from build123d import *

# Parameters (mm, degrees)
SKETCH_W            = 86.36
SKETCH_H            = 113.03
PAD_DEPTH           = 10
SKETCH001_R         = 1.6
POCKET_DEPTH        = 1
POCKET001_DEPTH     = 9
CHAMFER_SIZE        = 3
FILLET_R            = 6
FILLET_FACE23_R     = 1.6
POCKET002_DEPTH     = 9.001
POCKET002_FACE25_R  = 1.6
POCKET003_DEPTH     = 9.001
SKETCH003_R         = 2.8
POCKET005_DEPTH     = 4
POCKET006_DEPTH     = 10.001
POCKET006_FACE37_R  = 1.6
POCKET007_DEPTH     = 9.0010001
POCKET007_FACE6_R   = 1.6
POCKET008_DEPTH     = 4.5
CHAMFER001_SIZE     = 3
CHAMFER001_FACE10_W = 66.9783844647
CHAMFER001_FACE10_H = 4.5
POCKET009_DEPTH     = 2.5
CHAMFER002_SIZE     = 1


with BuildPart() as part:
    # Sketch → Pad (new body)
    with BuildSketch(Plane.XY):
        Rectangle(SKETCH_W, SKETCH_H)
    extrude(amount=PAD_DEPTH)

    # Sketch001 (on Face6 of Pad) → Pocket (cut)
    with BuildSketch(Plane.XY.offset(10)):
        with Locations((-39.37, -52.705)):
            Circle(SKETCH001_R)
        with Locations((39.37, -52.705)):
            Circle(SKETCH001_R)
        with Locations((39.37, 52.705)):
            Circle(SKETCH001_R)
    extrude(amount=-POCKET_DEPTH, mode=Mode.SUBTRACT)

    # Sketch002 (on Face5 of Pocket) → Pocket001 (cut)
    with BuildSketch(Plane.XY.offset(10)):
        with BuildLine():
            Line((-38.18, 56.515), (34.734927185, 56.515))
            ThreePointArc((34.734927185, 56.515), (33.7166110056, 50.695225665), (38.18, 46.8241922324))
            Line((38.18, -46.8241922324), (38.18, 46.8241922324))
            ThreePointArc((38.18, -46.8241922324), (35.1273593129, -48.4623593129), (33.4891922324, -51.515))
            Line((-33.4891922324, -51.515), (33.4891922324, -51.515))
            ThreePointArc((-33.4891922324, -51.515), (-35.1273593129, -48.4623593129), (-38.18, -46.8241922324))
            Line((-38.18, -46.8241922324), (-38.18, 56.515))
        make_face()
    extrude(amount=-POCKET001_DEPTH, mode=Mode.SUBTRACT)

    # Chamfer
    chamfer_edges = [part.edges().sort_by_distance(p)[0] for p in [
        (43.18, 0, 0),
        (0, -56.515, 0),
        (-43.18, 0, 0),
    ]]
    chamfer(chamfer_edges, length=CHAMFER_SIZE)

    # Fillet
    fillet_edges = [part.edges().sort_by_distance(p)[0] for p in [
        (43.18, 0, 3),
        (0, -56.515, 3),
        (-43.18, 0, 3),
    ]]
    fillet(fillet_edges, radius=FILLET_R)

    # Fillet Face23 → Pocket002 (cut, through all)
    with BuildSketch(Plane(origin=(39.37, 52.705, 9), x_dir=(0, 1, 0), z_dir=(0, 0, 1))):
        Circle(FILLET_FACE23_R)
    extrude(amount=-POCKET002_DEPTH, mode=Mode.SUBTRACT)

    # Pocket002 Face25 → Pocket003 (cut, through all)
    with BuildSketch(Plane(origin=(39.37, -52.705, 9), x_dir=(0, 1, 0), z_dir=(0, 0, 1))):
        Circle(POCKET002_FACE25_R)
    extrude(amount=-POCKET003_DEPTH, mode=Mode.SUBTRACT)

    # Sketch003 → Pocket005 (cut)
    with BuildSketch(Plane(origin=(0, 0, 0), x_dir=(1, 0, 0), z_dir=(0, 0, -1))):
        with Locations((-39.37, 52.705)):
            Circle(SKETCH003_R)
        with Locations((39.37, 52.705)):
            Circle(SKETCH003_R)
        with Locations((39.37, -52.705)):
            Circle(SKETCH003_R)
    extrude(amount=-POCKET005_DEPTH, mode=Mode.SUBTRACT)

    # Sketch004 (on Face4 of Pocket005) → Pocket006 (cut, through all)
    with BuildSketch(Plane(origin=(0, 0, 0), x_dir=(1, 0, 0), z_dir=(0, 0, -1))):
        Polygon((34.734927185, -56.515), (-43.18, -31.515), (-74.957912, -45.45311), (-56.152271, -90.823143), (38.876451, -98.385315), align=None)
    extrude(amount=-POCKET006_DEPTH, mode=Mode.SUBTRACT)

    # Pocket006 Face37 → Pocket007 (cut, through all)
    with BuildSketch(Plane(origin=(-39.37, -52.705, 9), x_dir=(0, 1, 0), z_dir=(0, 0, 1))):
        Circle(POCKET006_FACE37_R)
    extrude(amount=-POCKET007_DEPTH, mode=Mode.SUBTRACT)

    # Pocket007 Face6 → Pocket008 (cut)
    with BuildSketch(Plane(origin=(4.1610773178, -17.506602636, 10), x_dir=(0, 1, 0), z_dir=(0, 0, 1))):
        with BuildLine():
            Line((-39.008397364, 47.3410773178), (-39.008397364, -39.0189226822))
            Line((-39.008397364, -39.0189226822), (74.021602636, -39.0189226822))
            Line((74.021602636, -39.0189226822), (74.021602636, -30.5738498672))
            ThreePointArc((74.021602636, -30.5738498672), (68.201828301, -29.5555336878), (64.3307948684, -34.0189226822))
            Line((64.3307948684, -34.0189226822), (-29.3175895963, -34.0189226822))
            ThreePointArc((-29.3175895963, -34.0189226822), (-30.9557566768, -30.9662819951), (-34.008397364, -29.3281149145))
            Line((-34.008397364, -29.3281149145), (-34.008397364, 37.6502695502))
            ThreePointArc((-34.008397364, 37.6502695502), (-30.9557566768, 39.2884366307), (-29.3175895963, 42.3410773178))
            Line((-29.3175895963, 42.3410773178), (50.6259165271, 42.3410773178))
            Line((50.6259165271, 42.3410773178), (49.021602636, 47.3410773178))
            Line((49.021602636, 47.3410773178), (-39.008397364, 47.3410773178))
        make_face()
        with Locations((-35.198397364, -35.2089226822)):
            Circle(POCKET007_FACE6_R, mode=Mode.SUBTRACT)
        with Locations((70.211602636, -35.2089226822)):
            Circle(POCKET007_FACE6_R, mode=Mode.SUBTRACT)
        with Locations((-35.198397364, 43.5310773178)):
            Circle(POCKET007_FACE6_R, mode=Mode.SUBTRACT)
    extrude(amount=-POCKET008_DEPTH, mode=Mode.SUBTRACT)

    # Chamfer001
    chamfer001_edges = [part.edges().sort_by_distance(p)[0] for p in [
        (-38.18, -6.852439, 1),
        (38.18, 0, 1),
    ]]
    chamfer(chamfer001_edges, length=CHAMFER001_SIZE)

    # Chamfer001 Face10 → Pocket009 (cut)
    with BuildSketch(Plane(origin=(0, -51.515, 3.25), x_dir=(1, 0, 0), z_dir=(0, 1, 0))):
        Rectangle(CHAMFER001_FACE10_W, CHAMFER001_FACE10_H)
    extrude(amount=-POCKET009_DEPTH, mode=Mode.SUBTRACT)

    # Chamfer002
    chamfer002_edges = [part.edges().sort_by_distance(p)[0] for p in [
        (0, -54.015, 1),
    ]]
    chamfer(chamfer002_edges, length=CHAMFER002_SIZE)


solid = part.part
Here's how the part is built. I have some questions about the finished solid (model axes, mm). A direction names the side the tool comes from. Give positions to 0.01 mm unless a question says otherwise; leave off trailing zeros. Loops run counter-clockwise (first coordinate to the right, second up) from the corner with the lowest first, then second, coordinate; pieces in that order, holes last. Notation, with made-up numbers: (-0.5, 69) -> (11.5, 69) arc R11 ccw to (11.5, 88) -> close; hole circle Ø7 at (74, 53.25). An arc over 180 degrees is marked (long way). One line per item, written item: value.
Q1. Suppose I cut it at C-C on x = 14.5. Please give me the cut outline in (y, z) (3 decimals), then the cut area to 3 significant figures.
Answers follow:
outline: (-56.515, 5.485) arc R6 ccw to (-54.758, 1.243) -> (-53.515, 0) -> (50.022, 0) -> (50.022, 1) -> (-53.015, 1) -> (-54.015, 2) -> (-54.015, 5.5) -> (-56.515, 5.5) -> close
area: 113 mm^2
Q2. We'd pull the mould along X, two halves only. Please class faces 5 (the face through (37.15, -51, 2.42)), 6 (the face through (-12.698, 41.296, 0.496)), 7 (the face through (41, -17, 5.5)): pulls with the +X half, pulls with the -X half, needs draft (parallel to the pull), parting line crosses it, or undercut.
Answers follow:
face 5: undercut
face 6: pulls with the -X half
face 7: needs draft
Q3. If I drill on line 1 along Y through (x, z) = (39.37, 5) (3 decimals); line 2 along Y through (x, z) = (39.37, 1.55) (3 decimals); line 3 along X through (y, z) = (31.5, 5.15), over which ranges is the centre line in solid material (lowest first)?
Answers follow:
line 1: -56.495 to -54.305, -51.105 to 51.105, 54.305 to 56.515
line 2: -49.905 to 49.905, 55.505 to 56.515
line 3: -43.17 to -38.18, 38.18 to 43.17
Q4. I'm going to push flat-ended pins straight in: pin 1 Ø4 at (x, y) = (-39.37, -52.705) entering from +Z; pin 2 Ø1.1 at (x, z) = (-2, 3.5) entering from +Y (3 decimals); pin 3 Ø1.6 at (y, z) = (-25, 4.5) entering from +X; pin 4 Ø1.2 at (y, z) = (-10.5, 4.5) entering from -X. Where does each tip first touch, or does it pass through?
Answers follow:
pin 1: z = 5.5
pin 2: y = -54.015
pin 3: x = 43.18
pin 4: x = -43.17
Q5. On a 3-axis mill with a long thin cutter (end or side, diameter ignored), from which of +Z, -Z, +X, -X, +Y, -Y can I reach the whole of each face in a straight line? I mean faces 1 (the face through (36.573, 52.582, 1.972)), 2 (the face through (36.7, -0.68, 2.52)), 3 (the face through (33.688, 50.777, 3.281)), 4 (the face through (-34.58, -49.09, 3.28)). Say none if no direction works.
Answers follow:
face 1: -Z
face 2: +Z
face 3: +Z, -X
face 4: +Z, +Y
Q6. Suppose I cut it at B-B on x = -11.5. Please give me the cut outline in (y, z) (3 decimals).
Answers follow:
outline: (-56.515, 5.485) arc R6 ccw to (-54.758, 1.243) -> (-53.515, 0) -> (41.68, 0) -> (41.68, 1) -> (-53.015, 1) -> (-54.015, 2) -> (-54.015, 5.5) -> (-56.515, 5.5) -> close
